Geometry: final body of the model. Coordinates: model frame, mm. Coordinates: 2 decimals unless noted, no trailing zeros. Write each loop counter-clockwise with the first axis right and the second up, starting at its lowest first coordinate (ties: lowest second). Pieces come first, ordered by that corner, then holes. Notation, with made-up numbers: M 36.25,-20 L 63.25,-20 A20 ccw 63.25,-6 Z; hole C -4,-22 d7. An arc over 180 degrees is marked long. Write item = value, one per line. Start each with the question number.
Item 1: Pull-direction query (Z, two-part tool) for faces 1 (the cylindrical face through (-5.83, 179.896, 627.2)), 2 (the flat face through (-6, 214.67, 625)), 3 (the cylindrical face through (-5.67, 205.408, 631.115)), 4 (the cylindrical face through (-5.67, 205.408, 623.115)); classes: +Z half, -Z half, draft (parallel to the pull), parting line (faces both ways), or undercut.
Item 2: Section D-D on y = 189.5. Output: boundary loops of the cut face in (x, z), plus the area to 3 significant figures.
Item 3: Section C-C on y = 193.5. Output: boundary loops of the cut face in (x, z), plus the area to 3 significant figures.
Item 4: First-contact query: pin 1 Ø1.9 at (y, z) = (182.47, 614.23) entering from +X. Flat tip, straight axial feed; report the tip coordinate or a pass-through.
Item 5: Section A-A on y = 183.5. Output: boundary loops of the cut face in (x, z), plus the area to 3 significant figures.
Item 6: Ray query, L1, parallel to Z at x = -9.5, y = 204; L2, parallel to Y at x = -7.75, z = 614.25; L3, parallel to Y at x = -9.5, z = 624.75. Return the intervals inside material, ascending. Write a range as [from, to].
Item 7: Section B-B on x = -6.25. Output: boundary loops of the cut face in (y, z).
Autodesk Inventor part; units mm, degrees
ref_plane "YZ Plane" through (0, 0, 0) normal (1, 0, 0) x (0, 1, 0)
ref_plane "XZ Plane" through (0, 0, 0) normal (0, 1, 0) x (-1, 0, 0)
ref_plane "XY Plane" through (0, 0, 0) normal (0, 0, 1) x (1, 0, 0)
sketch "スケッチ1" plane through (0, 0, 0) normal (1, 0, 0) x (0, 1, 0)
  line L0 (214.6701, 659.5349) -> (214.6701, -648.4651)
  line L1 (214.6701, 627.3349) -> (194.6701, 627.3349)
  line L2 (194.6701, 659.5349) -> (194.6701, -648.4651)
  line L3 (194.6701, 23.5349) -> (214.6701, 23.5349)
  line L4 (194.6701, -648.4651) -> (214.6701, -648.4651)
  line L5 (194.6701, 659.5349) -> (214.6701, 659.5349)
  line L6 (179.6701, 611.4349) -> (207.4701, 611.4349)
  line L7 (207.4701, 611.4349) -> (207.4701, 627.3349)
  line L8 (207.4701, 627.3349) -> (179.6701, 627.3349)
  line L9 (179.6701, 627.3349) -> (179.6701, 611.4349)
  circle A0 centre (182.4701, 614.2349) radius 1.6
  circle A1 centre (204.6701, 624.5349) radius 1.6
  circle A2 centre (204.6701, 632.5349) radius 1.6
  line L10 (179.6701, 77.6349) -> (207.4701, 77.6349)
  line L11 (207.4701, 77.6349) -> (207.4701, 61.7349)
  line L12 (207.4701, 61.7349) -> (179.6701, 61.7349)
  line L13 (179.6701, 61.7349) -> (179.6701, 77.6349)
  circle A3 centre (182.4701, 74.8349) radius 1.5
  circle A4 centre (204.6701, 64.5349) radius 1.5
  circle A5 centre (204.6701, 56.5349) radius 1.5
  line L14 (194.6701, 637.5349) -> (214.6701, 637.5349)
  line L15 (207.4701, 611.4349) -> (214.6701, 611.4349)
  line L16 (214.6701, 611.4349) -> (214.6701, 637.5349)
  line L17 (194.6701, 637.5349) -> (179.6701, 627.3349)
  point P0 (0, 0)
  point P1 (-205.3299, -216.1317)
  dimension "d0" = 672
  dimension "d1" = 27.8
  dimension "d2" = 15.9
  dimension "d3" = 3.2
  dimension "d4" = 3.2
  dimension "d5" = 2.8
  dimension "d6" = 2.8
  dimension "d7" = 2.8
  dimension "d8" = 2.8
  dimension "d9" = 0
  dimension "d10" = 10
  dimension "d11" = 3.2
  dimension "d12" = 8
  dimension "d13" = 10
  dimension "d14" = 27
  dimension "d15" = 27.8
  dimension "d16" = 15.9
  dimension "d17" = 3
  dimension "d18" = 3
  dimension "d19" = 2.8
  dimension "d20" = 2.8
  dimension "d21" = 2.8
  dimension "d22" = 2.8
  dimension "d23" = 10
  dimension "d24" = 560
  dimension "d25" = 3
  dimension "d26" = 8
  dimension "d27" = 10
  dimension "d28" = 5
extrude "押し出し1" add sketch "スケッチ1" against normal blind 11.5 contours L0 L1 L2 L14 | L0 L15 L7 L1 | L2 L8 L17 | L7 L6 L2 L1 | L2 L6 L9 L8
fillet "フィレット1" radius 2 5 edges at (-5.75, 194.6701, 637.5349) (-5.75, 214.6701, 637.5349) (-5.75, 214.6701, 611.4349) (-5.75, 179.6701, 611.4349) (-5.75, 179.6701, 627.3349)
equation "\"d3\" = d11"
equation "\"d4\" = d11"
equation "\"d6\" = d5"
equation "\"d7\" = d5"
equation "\"d8\" = d5"
equation "\"d20\" = d19"
equation "\"d21\" = d19"
equation "\"d22\" = d19"
properties part number "dribl-v1-3DP-l-F-1" material "ABS プラスチック"
Responses:
q1.face_1 = +Z half
q1.face_2 = draft
q1.face_3 = undercut
q1.face_4 = undercut
q2.outline = M -11.5,611.43 L 0,611.43 L 0,634.02 L -11.5,634.02 Z
q2.area = 260 mm²
q3.outline = M -11.5,611.43 L 0,611.43 L 0,636.74 L -11.5,636.74 Z
q3.area = 291 mm²
q4.pin_1 = through
q5.outline = M -11.5,611.43 L 0,611.43 L 0,613.01 L -11.5,613.01 Z; M -11.5,615.46 L 0,615.46 L 0,629.94 L -11.5,629.94 Z
q5.area = 185 mm²
q6.L1 = [611.43, 623.08], [625.99, 631.08], [633.99, 637.53]
q6.L2 = [179.67, 180.87], [184.07, 214.67]
q6.L3 = [179.67, 203.08], [206.26, 214.67]
q7.outline = M 179.67,613.43 A2 ccw 181.67,611.43 L 212.67,611.43 A2 ccw 214.67,613.43 L 214.67,635.53 A2 ccw 212.67,637.53 L 195.29,637.53 A2 ccw 194.16,637.19 L 180.55,627.93 A2 ccw 179.67,626.28 Z; hole C 182.47,614.23 d3.2; hole C 204.67,624.53 d3.2; hole C 204.67,632.53 d3.2
